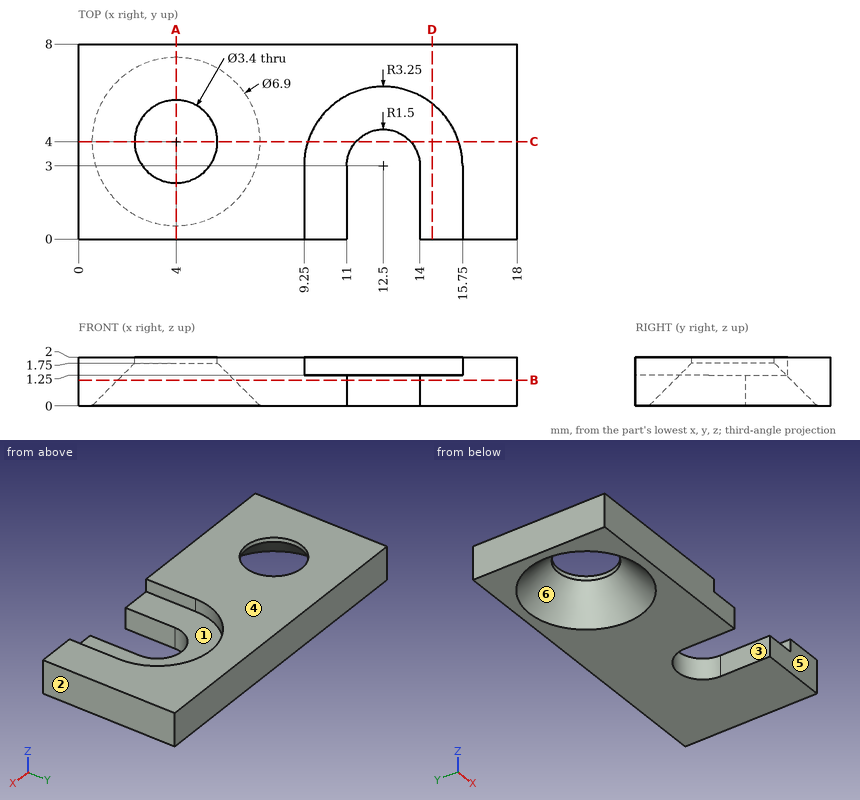
Design review of the part shown in the three views and the two pictorial views. Dimensions are in mm from the part's minimum x, y and z. A direction names the side the tool comes from. Round coordinates to 2 decimals unless told otherwise and drop trailing zeros. Loops run counter-clockwise (first coordinate to the right, second up) from the corner with the lowest first, then second, coordinate; pieces in that order, holes last. Notation, with made-up numbers: M 39,25 L 49,25 A22 ccw 49,60 Z; hole C -34,29.5 d6. An arc over 180 degrees is marked long. Write item = value, one per line.
Item 1: Machinability: for the marked faces 1, 2 and 3, which of the approach directions +Z, -Z, +X, -X, +Y, -Y give a long, thin tool a straight path to every point of the face, cutting with its end or side? Answer none if there is none.
Return value:
face_1 = +Z, -Y
face_2 = +Z, -Z, +X, +Y, -Y
face_3 = +Z, -Z, -Y
Item 2: Take a section at B-B on z = 1.05. Write out the cut boundary in (x, y).
Return value:
outline = M 0,0 L 11,0 L 11,3 A1.5 cw 14,3 L 14,0 L 18,0 L 18,8 L 0,8 Z; hole C 4,4 d4.8
Item 3: Take a section at D-D on x = 14.5. Write out the cut boundary in (y, z), then the cut area to 3 significant figures.
Return value:
outline = M 0,0 L 8,0 L 8,2 L 5.56,2 L 5.56,1.25 L 0,1.25 Z
area = 11.8 mm2
Item 4: Take a section at C-C on y = 4. Write out the cut boundary in (x, z), then the cut area to 3 significant figures.
Return value:
outline = M 0,0 L 0.55,0 L 2.3,1.75 L 2.3,2 L 0,2 Z; M 5.7,1.75 L 7.45,0 L 11.38,0 L 11.38,1.25 L 9.41,1.25 L 9.41,2 L 5.7,2 Z; M 13.62,0 L 18,0 L 18,2 L 15.59,2 L 15.59,1.25 L 13.62,1.25 Z
area = 18.7 mm2
Item 5: Take a section at A-A on x = 4. Write out the cut boundary in (y, z), then the cut area to 3 significant figures.
Return value:
outline = M 0,0 L 0.55,0 L 2.3,1.75 L 2.3,2 L 0,2 Z; M 5.7,1.75 L 7.45,0 L 8,0 L 8,2 L 5.7,2 Z
area = 6.14 mm2
Item 6: For line 1 (Y direction, x = 4, z = 1.95); line 2 (X direction, y = 2, z = 1.6); line 3 (X direction, y = 2.25, z = 0.25), list the stretches that pass through material, from the lowest coordinate up. Write a range as [from, to].
Return value:
line_1 = [0, 2.3], [5.7, 8]
line_2 = [0, 9.25], [15.75, 18]
line_3 = [0, 1.32], [6.68, 11], [14, 18]
Item 7: The part is to be moulded in two halves that separate along Y. For the marked faces 4, 5 and 6, say which applies: released by +Y, released by -Y, zero draft, split by the parting line, or undercut.
Return value:
face_4 = zero draft
face_5 = released by -Y
face_6 = undercut
